Autodesk Inventor part; units mm, degrees
ref_plane "YZ Plane" through (0, 0, 0) normal (1, 0, 0) x (0, 1, 0)
ref_plane "XZ Plane" through (0, 0, 0) normal (0, 1, 0) x (-1, 0, 0)
ref_plane "XY Plane" through (0, 0, 0) normal (0, 0, 1) x (1, 0, 0)
sketch "Sketch1" plane through (0, 0, 0) normal (0, 0, 1) x (1, 0, 0)
  line L0 (-102.5, -220) -> (102.5, -220)
  line L1 (102.5, -220) -> (102.5, 220)
  line L2 (102.5, 220) -> (-102.5, 220)
  line L3 (-102.5, 220) -> (-102.5, -220)
  line L4 (-102.5, -220) -> (102.5, 220) construction
  line L5 (102.5, -220) -> (-102.5, 220) construction
  line L6 (-96.5, 220) -> (-99.5, 220)
  line L7 (-99.5, 220) -> (-99.5, 0)
  line L8 (-99.5, 0) -> (-96.5, 0)
  line L9 (-96.5, 0) -> (-96.5, 220)
  line L10 (0, 220) -> (0, 0)
  line L11 (99.5, 220) -> (99.5, 0)
  line L12 (99.5, 0) -> (96.5, 0)
  line L13 (96.5, 0) -> (96.5, 220)
  dimension "d0" = 205
  dimension "d1" = 440
  dimension "d2" = 3
  dimension "d3" = 3
  dimension "d4" = 220
sketch "Sketch2" plane through (0, 0, 3) normal (0, 0, 1) x (1, 0, 0)
  line L0 (-96.5, 250) -> (96.5, 250)
  line L1 (96.5, 250) -> (96.5, 220)
  line L2 (96.5, 220) -> (-96.5, 220)
  line L3 (-96.5, 220) -> (-96.5, 250)
  line L4 (-96.5, 250) -> (96.5, 220) construction
  line L5 (96.5, 250) -> (-96.5, 220) construction
  line L6 (-96.5, 220) -> (96.5, 220)
  point P0 (0, 0)
  point P1 (0, 235)
  point P2 (0, 220)
  dimension "d6" = 30
extrude "Plate1" add sketch "Sketch1" along normal blind 3 contours L3 L2 L7 L8 L9 L13 L12 L11 L1 L0
sheet face with bend "Face2" sketch "Sketch2" thickness 3 toward (0, 0, -1) bend radius 3
bend "Bend1"
equation "\"d5\" = Thickness"
equation "\"d7\" = BendRadius"
equation "\"d8\" = BendReliefWidth"
equation "\"d10\" = MinimumRemnant"
equation "\"d9\" = BendReliefDepth"
equation "\"d11\" = TransitionRadius"
equation "\"BendRadius\" = Thickness"
equation "\"BendReliefWidth\" = Thickness"
equation "\"BendReliefDepth\" = 0.5 * Thickness"
equation "\"CornerReliefSize\" = 4 * Thickness"
equation "\"MinimumRemnant\" = 2 * Thickness"
equation "\"TransitionRadius\" = BendRadius"
equation "\"JacobiRadiusSize\" = BendRadius"
equation "\"GapSize\" = Thickness"
properties part number "Finishing Sheets .4 ( Front )  Acrylic" material "PMMA Plastic"
Can you work these out from the model? Positions are in its coordinate system, mm. Give positions to 0.01 mm unless a question says otherwise; leave off trailing zeros. Loops run counter-clockwise (first coordinate to the right, second up) from the corner with the lowest first, then second, coordinate; pieces in that order, holes last. Notation, with made-up numbers: (-17.5, -8.75) - (40.5, -8.75) arc R21 ccw to (40.5, 4.25) - close; hole circle Ø8 at (6.25, 22). An arc over 180 degrees is marked (long way). Return JSON: item names as keys, results as strings.
1. I'm going to push flat-ended pins straight in: pin 1 Ø0.9 at (x, z) = (-97.5, 2) entering from +Y; pin 2 Ø1.5 at (x, z) = (-101, 2) entering from +Y. Where does each tip first touch, or does it pass through?
Output values:
{"pin 1": "stops at y = 0", "pin 2": "stops at y = 220"}
2. I want a section at B-B on z = 0.5. Please give me the cut outline in (x, y).
Output values:
{"outline": "(-102.5, -220) - (102.5, -220) - (102.5, 220) - (99.5, 220) - (99.5, 0) - (96.5, 0) - (96.5, 250) - (-96.5, 250) - (-96.5, 0) - (-99.5, 0) - (-99.5, 220) - (-102.5, 220) - close"}
3. I want a section at A-A on y = 185. Please give me the cut outline in (x, z).
Output values:
{"outline": "(-102.5, 0) - (-99.5, 0) - (-99.5, 3) - (-102.5, 3) - close; (-96.5, 0) - (96.5, 0) - (96.5, 3) - (-96.5, 3) - close; (99.5, 0) - (102.5, 0) - (102.5, 3) - (99.5, 3) - close"}
4. If I drill on line 1 (X direction, y = 182, z = 2.65), over which ranges is the centre line in solid material (lowest first)?
Output values:
{"line 1": "x = -102.5 to -99.5, -96.5 to 96.5, 99.5 to 102.5"}
